from build123d import *

# Parameters (mm, degrees)
F0_R     = 38.1
F0_R_2   = 19.05
F1_DEPTH = 25.4
F2_W     = 25.4
F2_H     = 8.89
F3_ANGLE = 180
F4_R     = 3.81
F5_SIZE  = 3.81


with BuildPart() as f1:
    # F0 (on Front) → F1 (new body)
    with BuildSketch(Plane.XZ):
        Circle(F0_R)
        Circle(F0_R_2, mode=Mode.SUBTRACT)
    extrude(amount=F1_DEPTH)

    # F2 (on face) → F3 (revolve)
    with BuildSketch(Plane.XZ.offset(25.4)):
        with Locations((0.5661081523, 24.5059088439)):
            Rectangle(F2_W, F2_H)
    revolve(axis=Axis((-5.3780302405, -25.4, 0), (1, 0, 0)), revolution_arc=F3_ANGLE)

    # F4
    f4_edges = [f1.edges().sort_by_distance(p)[0] for p in [
        (13.266108, -54.350909, 0),
        (-12.133892, -54.350909, 0),
        (13.266108, -45.460909, 0),
        (-12.133892, -45.460909, 0),
    ]]
    fillet(f4_edges, radius=F4_R)

    # F5
    f5_edges = [f1.edges().sort_by_distance(p)[0] for p in [
        (-38.1, -25.4, 0),
        (-38.1, 0, 0),
    ]]
    chamfer(f5_edges, length=F5_SIZE)


solid = f1.part
Check sheet for the modelled part. Datum: model origin and axes. Units: mm. A direction names the side the tool comes from. Give positions to 0.01 mm unless a question says otherwise; leave off trailing zeros. Write each loop counter-clockwise with the first axis right and the second up, starting at its lowest first coordinate (ties: lowest second). Pieces come first, ordered by that corner, then holes. Notation, with made-up numbers: M -34.5,20.25 L -8.5,20.25 A20 ccw -8.5,39.25 Z; hole C 26,28.5 d10. An arc over 180 degrees is marked long. Use one line per item in the form item = value.
(1) Tool access check on faces 1 (the flat face through (-12.134, -49.2, -3.6)), 2 (the flat face through (13.266, -49.2, -3.6)), 3 (the cylindrical face through (-15.12, -12.52, -11.59)). Record the directions out of +Z, -Z, +X, -X, +Y, -Y that give a thin tool (end or side, any length) a straight path to the whole face; none if there is none.
Answer block:
face_1 = +Z, -Z, -X, -Y
face_2 = +Z, -Z, +X, -Y
face_3 = +Y
(2) Material ranges on line 1 along X through (y, z) = (-16, -0.5); line 2 along Z through (x, y) = (0, -8.5); line 3 along Y through (x, z) = (-5, -30), recorded low to high.
Answer block:
line_1 = -38.1 to -19.04, 19.04 to 38.1
line_2 = -38.1 to -19.05, 19.05 to 38.1
line_3 = -25.4 to 0
(3) Draft check along Y on faces 4 (the cylindrical face through (0.691, -54.344, 0.637)), 5 (the cylindrical face through (0.691, -45.456, 0.441)), 6 (the flat face through (15, 0, -15)). Enter one of: pulls with the +Y half, pulls with the -Y half, needs draft (parallel to the pull), parting line crosses it, or undercut.
Answer block:
face_4 = pulls with the -Y half
face_5 = undercut
face_6 = pulls with the +Y half
(4) Section check B-B on x = 0. Record the boundary of the cut face in (y, z), plus the area to 3 significant figures.
Answer block:
outline = M -25.4,-34.29 L -21.59,-38.1 L -3.81,-38.1 L 0,-34.29 L 0,-19.05 L -25.4,-19.05 L -25.4,-20.06 A20.06 cw -25.4,20.06 L -25.4,19.05 L 0,19.05 L 0,34.29 L -3.81,38.1 L -21.59,38.1 L -25.4,34.29 L -25.4,28.95 A28.95 ccw -25.4,-28.95 Z
area = 1,620 mm2
(5) Section check C-C on z = -17.5. State how many separate pieces and enclosed holes the cut face has, plus the area to 3 significant figures.
Answer block:
separate_pieces = 3
enclosed_holes = 0
area = 1,620 mm2
(6) Depth check by flat-ended pin: P1, Ø5, axis at x = 14, y = -24, coming from the +Z side; P2, Ø2, axis at y = -17, z = -22.5, coming from the -X side; P3, Ø1, axis at y = -39.5, z = -20, coming from the -X side. Enter the tip coordinate at first touch or a pass-through.
Answer block:
P1 = 35.7
P2 = -31.45
P3 = -12.13
(7) Section check A-A on z = 0. Record the boundary of the cut face in (x, y).
Answer block:
outline = M -38.1,-21.59 L -34.29,-25.4 L -19.05,-25.4 L -19.05,0 L -34.29,0 L -38.1,-3.81 Z; M -12.13,-50.54 A3.81 ccw -8.32,-54.35 L 9.46,-54.35 A3.81 ccw 13.27,-50.54 L 13.27,-49.27 A3.81 ccw 9.46,-45.46 L -8.32,-45.46 A3.81 ccw -12.13,-49.27 Z; M 19.05,-25.4 L 34.29,-25.4 L 38.1,-21.59 L 38.1,-3.81 L 34.29,0 L 19.05,0 Z
